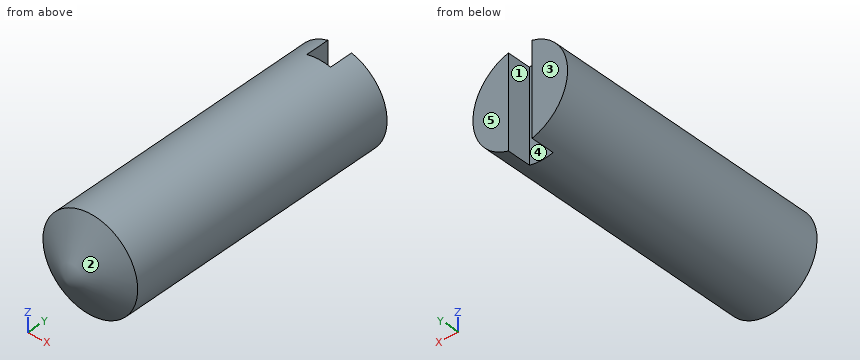
from build123d import *

# Parameters (mm, degrees)
SKETCH1_R           = 2
BOSS_EXTRUDE1_DEPTH = 13
CHAMFER1_SIZE       = 2
CHAMFER1_SIZE2      = 1.154700538
SKETCH2_W           = 1
SKETCH2_H           = 4.464568748
CUT_EXTRUDE1_DEPTH  = 1


with BuildPart() as part:
    # Sketch1 → Boss-Extrude1 (new body)
    with BuildSketch(Plane(origin=(0, 0, 0), x_dir=(1, 0, 0), z_dir=(0, 1, 0))):
        with Locations(Location((0, 0, 0), (0, 0, 90))):
            Circle(SKETCH1_R)
    extrude(amount=BOSS_EXTRUDE1_DEPTH)

    # Chamfer1
    chamfer1_edges = [part.edges().sort_by_distance(p)[0] for p in [
        (0, 0, 2),
    ]]
    chamfer1_side = [part.faces().sort_by_distance(p)[0] for p in [
        (0, 0, 0),
    ]]
    chamfer(chamfer1_edges, length=CHAMFER1_SIZE, length2=CHAMFER1_SIZE2, reference=chamfer1_side[0])

    # Sketch2 → Cut-Extrude1 (cut)
    with BuildSketch(Plane(origin=(0, 13, 0), x_dir=(1, 0, 0), z_dir=(0, 1, 0))):
        with Locations((0, -0.081308371)):
            Rectangle(SKETCH2_W, SKETCH2_H)
    extrude(amount=-CUT_EXTRUDE1_DEPTH, mode=Mode.SUBTRACT)


solid = part.part
Verification items for the finished model (mm, model axes). Face numbers are marked on the shaded views. A direction names the side the tool comes from. Give positions to 0.01 mm unless a question says otherwise; leave off trailing zeros. Loops run counter-clockwise (first coordinate to the right, second up) from the corner with the lowest first, then second, coordinate; pieces in that order, holes last.
1) Depth check by flat-ended pin: pin 1 Ø0.5 at (y, z) = (12.5, 0.5) entering from -X; pin 2 Ø0.5 at (y, z) = (12.5, -0.5) entering from +X. Enter the tip coordinate at first touch or a pass-through.
2) Set-up check for the marked faces 4 and 5: record each of +Z, -Z, +X, -X, +Y, -Y from which the full face is reachable in a straight line by a thin tool's end or side.
3) Draft check along X on the marked faces 1, 2 and 3. Enter one of: pulls with the +X half, pulls with the -X half, needs draft (parallel to the pull), parting line crosses it, or undercut.
4) Thickness scan on line 1 along X through (y, z) = (10.5, -0.5); line 2 along Y through (x, z) = (-1.45, -1); line 3 along Z through (x, y) = (1.2, 1.25). Record the ranges inside material, lowest first.
5) Sectioned sample at A-A, the plane y = 11.25. Enter the section's corners in (x, z), then the cut area to 3 significant figures.
Answers:
1. pin 1: stops at x = -1.98
1. pin 2: stops at x = 1.98
2. face 4: +Z, -Z, +Y
2. face 5: +Z, -Z, +X, -X, +Y
3. face 1: undercut
3. face 2: parting line crosses it
3. face 3: needs draft
4. line 1: x = -1.94 to 1.94
4. line 2: y = 1.02 to 13
4. line 3: z = -1.6 to 1.6
5. outline: circle Ø4 at (0, 0)
5. area: 12.6 mm2
